Can you work these out from the model? Positions are in its coordinate system, mm. A direction names the side the tool comes from. Coordinates: 2 decimals unless noted, no trailing zeros. Order: outer loops, then holes, each group sorted by start corner. A loop starts at its lowest first (then second) coordinate and runs counter-clockwise, first axis right, second up. Notation, with made-up numbers: (35, 15.25) -> (56, 15.25) arc R17 cw to (56, 30.25) -> close; hole circle Ø2 at (30, 45). An arc over 180 degrees is marked (long way). Answer as a JSON object with one key per item and string values. Group by question number.
(1) For pin 1 (10 mm diameter, centred on x = -200, z = -200, fed in from -Y); pin 2 (7 mm diameter, centred on x = -200, z = 200, fed in from +Y); pin 3 (22 mm diameter, centred on x = -135, y = 12.5, fed in from +Z), each with a flat end and sliding along its axis, tell me the tip position at first contact or that it passes through.
(2) If we mould it in two halves opening along Z, with no side actions, what happens to faces 1 (the flat face through (10, 20, -349)), 2 (the flat face through (10, -15, -425)), 3 (the flat face through (-10, -45, 6))? For each: pulls with the +Z half, pulls with the -Z half, needs draft (parallel to the pull), parting line crosses it, or undercut.
(3) Which directions (+Z, -Z, +X, -X, +Y, -Y) give clear straight access to the entire face, cutting with the end or side of a thin tool? Please do faces 4 (the flat face through (-10, 0, 80)), 5 (the flat face through (730, -23, -6)).
(4) I want a section at A-A, the plane z = 310.5. List the corners of the cut face in (x, y) for me, plus the area to 4 significant figures.
(5) I need wall thicknesses on line 1 (Z direction, x = 200, y = -2); line 2 (X direction, y = -3, z = 200); line 3 (Y direction, x = -221.5, z = -227.5). Which ranges of each line are inside material? Lowest first, please.
(6) I want a section at B-B, the plane x = 472.5. List the corners of the cut face in (y, z) for me.
from build123d import *

# Parameters (mm, degrees)
F0_W     = 1460
F0_H     = 850
F1_DEPTH = 50
F2_W     = 1410
F2_H     = 800
F3_DEPTH = 5
F5_D     = 6.3
F5_DEPTH = 5
F5_TIP   = 1.8927109499
F4_W     = 1460
F4_H     = 150
F6_DEPTH = 20


with BuildPart() as f1:
    # F0 (on Front) → F1 (new body)
    with BuildSketch(Plane.XZ):
        Rectangle(F0_W, F0_H)
    extrude(amount=F1_DEPTH)

    # F2 (on face) → F3 (cut)
    with BuildSketch(Plane.XZ.offset(50)):
        Rectangle(F2_W, F2_H)
    extrude(amount=-F3_DEPTH, mode=Mode.SUBTRACT)

    # F5
    with Locations(Plane(origin=(0, 0, 0), x_dir=(-1, 0, 0), z_dir=(0, 1, 0))):
        with Locations((-200, 200), (200, 200), (200, -200), (-200, -200)):
            Hole(F5_D / 2, depth=F5_DEPTH)
            with Locations((0, 0, -(F5_DEPTH + F5_TIP / 2))):  # 118° drill point
                Cone(0, F5_D / 2, F5_TIP, mode=Mode.SUBTRACT)

    # F4 (on face) → F6 (join)
    with BuildSketch(Plane(origin=(0, 0, 0), x_dir=(-1, 0, 0), z_dir=(0, 1, 0))):
        with Locations((0, -350)):
            Rectangle(F4_W, F4_H)
    extrude(amount=F6_DEPTH)


solid = f1.part
Computed values:
{
 "1": {"pin 1": "stops at y = -45", "pin 2": "stops at y = 0", "pin 3": "stops at z = -275"},
 "2": {"face 1": "needs draft", "face 2": "pulls with the -Z half", "face 3": "undercut"},
 "3": {"face 4": "+Z, +X, -X, +Y", "face 5": "+Z, -Z, +X, +Y, -Y"},
 "4": {"outline": "(-730, -50) -> (-705, -50) -> (-705, -45) -> (705, -45) -> (705, -50) -> (730, -50) -> (730, 0) -> (-730, 0) -> close", "area": "65,950 mm2"},
 "5": {"line 1": "z = -425 to -203.15, -196.85 to 196.85, 203.15 to 425", "line 2": "x = -730 to -203.15, -196.85 to 196.85, 203.15 to 730", "line 3": "y = -45 to 0"},
 "6": {"outline": "(-50, -425) -> (20, -425) -> (20, -275) -> (0, -275) -> (0, 425) -> (-50, 425) -> (-50, 400) -> (-45, 400) -> (-45, -400) -> (-50, -400) -> close"}
}
